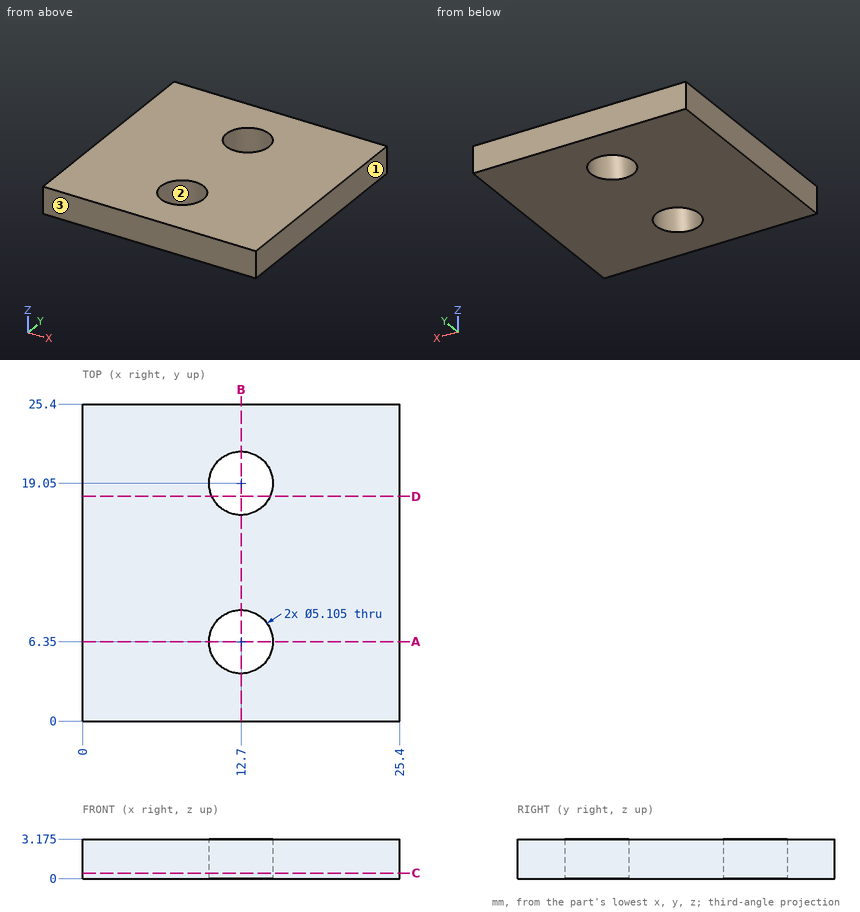
For this review, use the dimensioned drawing (mm, ordinates from the lowest corner) and the shaded views. Round coordinates to 2 decimals unless told otherwise and drop trailing zeros. Write each loop counter-clockwise with the first axis right and the second up, starting at its lowest first coordinate (ties: lowest second). Pieces come first, ordered by that corner, then holes. Notation, with made-up numbers: (40.5, -34.75) -> (98.5, -34.75) arc R28 ccw to (98.5, 3.25) -> close; hole circle Ø6 at (-3.5, 60). An arc over 180 degrees is marked (long way). Use CSV: the item, a comma, the result in double quotes.
Q1. Mouldability with a two-part tool opening along Y and no side actions: class the marked faces 1, 2 and 3 as released by +Y, released by -Y, zero draft, split by the parting line, or undercut.
Checks:
face 1,"zero draft"
face 2,"undercut"
face 3,"released by -Y"
Q2. To check wall thickness, follow probe 1 along Y at (x, z) = (12.7, 1.95); probe 2 along Y at (x, z) = (14.75, 2.5); probe 3 along X at (y, z) = (5.75, 1.15). State the ranges of each line that lie inside material, in increasing order. Write a range as [from, to].
Checks:
probe 1,"[0, 3.8], [8.9, 16.5], [21.6, 25.4]"
probe 2,"[0, 4.83], [7.87, 17.53], [20.57, 25.4]"
probe 3,"[0, 10.22], [15.18, 25.4]"
Q3. Consider section A-A (y = 6.35). Give the boundary of the cut face in (x, z) (1 decimal).
Checks:
outline,"(0, 0) -> (10.1, 0) -> (10.1, 3.2) -> (0, 3.2) -> close; (15.3, 0) -> (25.4, 0) -> (25.4, 3.2) -> (15.3, 3.2) -> close"
Q4. Consider section C-C (z = 0.45). State how many separate pieces and enclosed holes the cut face has, then the cut area to 3 significant figures.
Checks:
separate pieces,"1"
enclosed holes,"2"
area,"604 mm²"
Q5. Consider section B-B (x = 12.7). Give the boundary of the cut face in (y, z) (1 decimal).
Checks:
outline,"(0, 0) -> (3.8, 0) -> (3.8, 3.2) -> (0, 3.2) -> close; (8.9, 0) -> (16.5, 0) -> (16.5, 3.2) -> (8.9, 3.2) -> close; (21.6, 0) -> (25.4, 0) -> (25.4, 3.2) -> (21.6, 3.2) -> close"
Q6. Consider section D-D (y = 18). Give the boundary of the cut face in (x, z) (1 decimal).
Checks:
outline,"(0, 0) -> (10.4, 0) -> (10.4, 3.2) -> (0, 3.2) -> close; (15, 0) -> (25.4, 0) -> (25.4, 3.2) -> (15, 3.2) -> close"
